Geometry check sheet. Reference: the model listing, model coordinates, mm. Coordinates: 2 decimals unless noted, no trailing zeros. Write each loop counter-clockwise with the first axis right and the second up, starting at its lowest first coordinate (ties: lowest second). Pieces come first, ordered by that corner, then holes. Notation, with made-up numbers: (54, 19.25) -> (74, 19.25) arc R22 cw to (74, 45.25) -> close; hole circle Ø7 at (-15.5, 64). An arc over 180 degrees is marked (long way). Answer in a Markdown table with one row per item. Add a question column.
Q1. Section check C-C, the plane x = 1.2. Record the boundary of the cut face in (y, z) (3 decimals).
Q2. Section check D-D, the plane y = 17. Record the boundary of the cut face in (x, z), and give its area (3 significant figures).
Q3. Thickness scan on line 1 (Y direction, x = 0, z = 0) (3 decimals); line 2 (Y direction, x = -0.75, z = -2.5); line 3 (Z direction, x = 1.2, y = 35.5). Record the ranges inside material, lowest first.
Q4. Gauge pin test, flat ends, axial feed: P1, Ø1, axis at x = -1.5, y = 23, coming from the +Z side; P2, Ø4, axis at y = 10, z = 8.5, coming from the -X side (3 decimals); P3, Ø1.5, axis at x = 1.5, y = 10, coming from the +Z side. Record the tip position at first contact, or that the pin passes through.
Q5. Section check A-A, the plane z = 0. Record the boundary of the cut face in (x, y) (3 decimals).
Q6. Section check B-B, the plane y = 34.5. Record the boundary of the cut face in (x, z).
Q7. Release check for a two-part mould opening along Y. For faces 1 (the face through (0.035, 20.855, -13.365)), 2 (the face through (0.04, 15.87, 0.32)), 3 (the face through (-0.035, 43.832, 0.651)) record: pulls with the +Y half, pulls with the -Y half, needs draft (parallel to the pull), parting line crosses it, or undercut.
```python
from build123d import *

# Parameters (mm, degrees)
SKETCH2_R           = 5
BOSS_EXTRUDE1_DEPTH = 2.5


with BuildPart() as part:
    # Sketch2 → Boss-Extrude1 (new, symmetric)
    with BuildSketch(Plane(origin=(0, 0, 0), x_dir=(0, 0, -1), z_dir=(1, 0, 0))):
        with BuildLine():
            Line((-10.913166227, 40.254421222), (-15.749683077, 1.990755627))
            ThreePointArc((-15.749683077, 1.990755627), (0, 15.875), (15.749683077, 1.990755627))
            Line((15.749683077, 1.990755627), (10.913166227, 40.254421222))
            ThreePointArc((10.913166227, 40.254421222), (0, 49.875), (-10.913166227, 40.254421222))
        make_face()
        with Locations((0, 38.875)):
            Circle(SKETCH2_R, mode=Mode.SUBTRACT)
    extrude(amount=BOSS_EXTRUDE1_DEPTH, both=True)


solid = part.part
```
Calculated:
| question | item | result |
|---|---|---|
| 1 | outline | (1.991, -15.75) -> (40.254, -10.913) arc R11 ccw to (40.254, 10.913) -> (1.991, 15.75) arc R15.875 cw to start; hole circle Ø10 at (38.875, 0) |
| 2 | outline | (-2.5, -13.85) -> (2.5, -13.85) -> (2.5, 13.85) -> (-2.5, 13.85) -> close |
| 2 | area | 139 mm² |
| 3 | line 1 | y = 15.875 to 33.875, 43.875 to 49.875 |
| 3 | line 2 | y = 15.68 to 34.54, 43.21 to 49.59 |
| 3 | line 3 | z = -11.51 to -3.69, 3.69 to 11.51 |
| 4 | P1 | stops at z = 13.16 |
| 4 | P2 | passes through |
| 4 | P3 | stops at z = 14.83 |
| 5 | outline | (-2.5, 15.875) -> (2.5, 15.875) -> (2.5, 33.875) -> (-2.5, 33.875) -> close; (-2.5, 43.875) -> (2.5, 43.875) -> (2.5, 49.875) -> (-2.5, 49.875) -> close |
| 6 | outline | (-2.5, -11.64) -> (2.5, -11.64) -> (2.5, -2.42) -> (-2.5, -2.42) -> close; (-2.5, 2.42) -> (2.5, 2.42) -> (2.5, 11.64) -> (-2.5, 11.64) -> close |
| 7 | face 1 | pulls with the +Y half |
| 7 | face 2 | pulls with the -Y half |
| 7 | face 3 | undercut |
